```python
from build123d import *

# Parameters (mm, degrees)
SKETCH2_W           = 10
SKETCH2_H           = 14.768412439
BOSS_EXTRUDE1_DEPTH = 5
BOSS_EXTRUDE4_DEPTH = 10
SKETCH9_W           = 10
SKETCH9_H           = 3.18
SKETCH9_H_2         = 3.888412439
CUT_EXTRUDE3_DEPTH  = 5
BOSS_EXTRUDE5_DEPTH = 7.7
SKETCH12_R          = 0.75
BOSS_EXTRUDE7_DEPTH = 2.75
FILLET1_R           = 2.5


with BuildPart() as part:
    # Sketch2 → Boss-Extrude1 (new body)
    with BuildSketch(Plane.XY):
        with Locations((0, 1.566049366)):
            Rectangle(SKETCH2_W, SKETCH2_H)
    extrude(amount=BOSS_EXTRUDE1_DEPTH)

    # Sketch8 → Boss-Extrude4 (add)
    with BuildSketch(Plane.ZY.offset(5)):
        Polygon((-0.15, 5.770255585), (0, 5.770255585), (0, 4.070255585), (-0.15, 4.070255585), (-2.137867966, 4.070255585), (-3.402081528, 5.334469147), (-2.2, 6.536550675), (-1.43370491, 5.770255585), align=None)
        Polygon((-0.15, -1.929744415), (0, -1.929744415), (0, -0.229744415), (-0.15, -0.229744415), (-1.43370491, -0.229744415), (-2.2, 0.536550675), (-3.402081528, -0.665530853), (-2.137867966, -1.929744415), align=None)
    extrude(amount=-BOSS_EXTRUDE4_DEPTH)

    # Sketch9 → Cut-Extrude3 (cut)
    with BuildSketch(Plane(origin=(0, 0, 0), x_dir=(-1, 0, 0), z_dir=(0, 0, -1))):
        with Locations((0, 7.360255585)):
            Rectangle(SKETCH9_W, SKETCH9_H)
        with Locations((0, -3.873950635)):
            Rectangle(SKETCH9_W, SKETCH9_H_2)
    extrude(amount=-CUT_EXTRUDE3_DEPTH, mode=Mode.SUBTRACT)

    # Sketch10 → Boss-Extrude5 (add)
    with BuildSketch(Plane(origin=(0, 5.770255585, 0), x_dir=(1, 0, 0), z_dir=(0, 1, 0))):
        Polygon((-5, -5), (-5, -10.5), (1.352445729, -55.7), (6.352445729, -55.7), (6.352445729, -49.2), (5, -14), (5, -5), align=None)
    extrude(amount=-BOSS_EXTRUDE5_DEPTH)

    # Sketch12 → Boss-Extrude7 (add)
    with BuildSketch(Plane.XY):
        with BuildLine():
            Line((5, 5.770255585), (8.5, 5.770255585))
            ThreePointArc((8.5, 5.770255585), (12.35, 1.920255585), (8.5, -1.929744415))
            Line((8.5, -1.929744415), (5, -1.929744415))
            Line((5, -1.929744415), (5, 5.770255585))
        make_face()
        with Locations((8.5, 1.920255585)):
            Circle(SKETCH12_R, mode=Mode.SUBTRACT)
    extrude(amount=BOSS_EXTRUDE7_DEPTH)

    # Fillet1
    fillet1_edges = [part.edges().sort_by_distance(p)[0] for p in [
        (6.352445729, 1.920255585, 49.2),
        (5, 1.920255585, 14),
        (1.352445729, 1.920255585, 55.7),
        (6.352445729, 1.920255585, 55.7),
    ]]
    fillet(fillet1_edges, radius=FILLET1_R)


solid = part.part
```
The model under review builds one solid part; all positions refer to its coordinate system, in mm. A direction names the side the tool comes from. Round coordinates to 2 decimals unless told otherwise and drop trailing zeros. Write each loop counter-clockwise with the first axis right and the second up, starting at its lowest first coordinate (ties: lowest second). Pieces come first, ordered by that corner, then holes. Notation, with made-up numbers: M 26.25,39.25 L 81.25,39.25 A21 ccw 81.25,58.25 Z; hole C 24,85 d1. An arc over 180 degrees is marked long. Use CSV: the item, a comma, the result in double quotes. Start each with the question number.
(1) Tool access review of faces 1 (the face through (9, 1, 2.75)), 2 (the face through (0, -0.23, -1)), 3 (the face through (2, 5.77, 20)), 4 (the face through (6.352, 2, 51)), 5 (the face through (5, -1, -2)): name each direction out of +Z, -Z, +X, -X, +Y, -Y from which nothing blocks a thin tool from reaching the whole face with its end or side.
(2) We need section B-B, the plane z = 6. State the section outline as (x, y) points.
(3) We need section A-A, the plane x = 2.25. State the section outline as (y, z) points.
(4) Clearance check with flat-ended pins moving along their axes: P1, Ø2.5, axis at y = -1, z = -2, coming from the +X side; P2, Ø1.7, axis at x = 8.5, y = 1.92, coming from the +Z side; P3, Ø4.5, axis at y = 2.5, z = 50.5, coming from the +X side. State where each tip first meets the part, or that it passes through.
(5) We need section C-C, the plane z = 32.5. State the section outline as (x, y) points.
(6) For line 1 along Y through (x, z) = (8.5, 0.6); line 2 along Z through (x, y) = (7.25, -0.25); line 3 along Y through (x, z) = (8, 1), list the stretches that pass through material, from the lowest coordinate up.
(7) The part is to be moulded in two halves that separate along Z. For faces 6 (the face through (-0.07, -0.056, -2.793)), 7 (the face through (-2.017, 1.974, 31.723)), 8 (the face through (5, 2, 8)), say which applies: +Z half, -Z half, draft (parallel to the pull), parting line (faces both ways), or undercut.
Findings:
1,face 1,"+X, +Y, -Y"
1,face 2,"+X, -X"
1,face 3,"+Z, +X, -X, +Y"
1,face 4,"+Z, +X, +Y, -Y"
1,face 5,"-Z, +X, +Y, -Y"
2,outline,"M -5,-1.93 L 5,-1.93 L 5,5.77 L -5,5.77 Z"
3,outline,"M -1.93,-2.14 L -0.67,-3.4 L 0.54,-2.2 L -0.23,-1.43 L -0.23,0 L 4.07,0 L 4.07,-2.14 L 5.33,-3.4 L 6.54,-2.2 L 5.77,-1.43 L 5.77,55.35 L -1.93,55.35 Z"
4,P1,"x = 5"
4,P2,"z = 2.75"
4,P3,"x = 6.35"
5,outline,"M -1.91,-1.93 L 5.71,-1.93 L 5.71,5.77 L -1.91,5.77 Z"
6,line 1,"-1.93 to 1.17, 2.67 to 5.77"
6,line 2,"0 to 2.75"
6,line 3,"-1.93 to 1.36, 2.48 to 5.77"
7,face 6,"-Z half"
7,face 7,"+Z half"
7,face 8,"undercut"
